from build123d import *

# Parameters (mm, degrees)
F1_DEPTH  = 63.5
F3_DEPTH  = 7.9375
F5_DEPTH  = 7.9375
F7_DEPTH  = 7.9375
F8_R      = 6.35
F9_R      = 9.92251
F10_DEPTH = 88.901
F11_R     = 10.3251
F12_DEPTH = 7.9385


with BuildPart() as f1:
    # F0 (on Right) → F1 (new body)
    with BuildSketch(Plane.YZ):
        with BuildLine():
            Line((-36.5125, 44.45), (-44.45, 44.45))
            Line((-44.45, 44.45), (-44.45, 12.7))
            ThreePointArc((-44.45, 12.7), (-40.7302561211, 3.7197438789), (-31.75, 0))
            Line((-31.75, 0), (0, 0))
            Line((0, 0), (0, 7.9375))
            Line((0, 7.9375), (-31.75, 7.9375))
            ThreePointArc((-31.75, 7.9375), (-35.1175960454, 9.3324039546), (-36.5125, 12.7))
            Line((-36.5125, 12.7), (-36.5125, 44.45))
        make_face()
        with BuildLine():
            Line((0, 7.9375), (0, 0))
            Line((0, 0), (31.75, 0))
            ThreePointArc((31.75, 0), (40.7302561211, 3.7197438789), (44.45, 12.7))
            Line((44.45, 12.7), (44.45, 44.45))
            Line((44.45, 44.45), (36.5125, 44.45))
            Line((36.5125, 44.45), (36.5125, 12.7))
            ThreePointArc((36.5125, 12.7), (35.1175960454, 9.3324039546), (31.75, 7.9375))
            Line((31.75, 7.9375), (0, 7.9375))
        make_face()
    extrude(amount=F1_DEPTH)

    # F2 (on face) → F3 (join, through all)
    with BuildSketch(Plane.XZ.offset(44.45)):
        with BuildLine():
            Line((0, 44.45), (63.5, 44.45))
            ThreePointArc((63.5, 44.45), (31.75, 76.2), (0, 44.45))
        make_face()
    extrude(amount=-F3_DEPTH)

    # F4 (on face) → F5 (join, through all)
    with BuildSketch(Plane(origin=(0, 44.45, 0), x_dir=(-1, 0, 0), z_dir=(0, 1, 0))):
        with BuildLine():
            ThreePointArc((0, 44.45), (-31.75, 76.2), (-63.5, 44.45))
            Line((-63.5, 44.45), (0, 44.45))
        make_face()
    extrude(amount=-F5_DEPTH)

    # F6 (on face) → F7 (join, through all)
    with BuildSketch(Plane(origin=(0, 0, 0), x_dir=(1, 0, 0), z_dir=(0, 0, -1))):
        with BuildLine():
            Line((63.5, 22.225), (63.5, -22.225))
            Line((63.5, -22.225), (117.475, -22.225))
            ThreePointArc((117.475, -22.225), (133.1904482119, -15.7154482119), (139.7, 0))
            ThreePointArc((139.7, 0), (133.1904482119, 15.7154482119), (117.475, 22.225))
            Line((117.475, 22.225), (63.5, 22.225))
        make_face()
    extrude(amount=-F7_DEPTH)

    # F8
    f8_edges = [f1.edges().sort_by_distance(p)[0] for p in [
        (63.5, -22.225, 3.96875),
        (63.5, 22.225, 3.96875),
    ]]
    fillet(f8_edges, radius=F8_R)

    # F9 (on face) → F10 (cut, through all)
    with BuildSketch(Plane.XZ.offset(44.45)):
        with Locations((31.75, 44.45)):
            Circle(F9_R)
    extrude(amount=-F10_DEPTH, mode=Mode.SUBTRACT)

    # F11 (on face) → F12 (cut, through all)
    with BuildSketch(Plane.XY.offset(7.9375)):
        with Locations((117.475, 0)):
            Circle(F11_R)
        with Locations((79.375, 0)):
            Circle(F11_R)
    extrude(amount=-F12_DEPTH, mode=Mode.SUBTRACT)


solid = f1.part
Read the model definition and answer for the solid it produces. Units are mm, in the model's axes. A direction names the side the tool comes from. Give positions to 0.01 mm unless a question says otherwise; leave off trailing zeros. Write each loop counter-clockwise with the first axis right and the second up, starting at its lowest first coordinate (ties: lowest second). Pieces come first, ordered by that corner, then holes. Notation, with made-up numbers: (60, -7) - (80, -7) arc R23 ccw to (80, 21) - close; hole circle Ø4 at (69, 56.5). An arc over 180 degrees is marked (long way). Return JSON: item names as keys, results as strings.
Q1. A cutting plane is placed at B-B, the plane x = 31.75. Count the separate pieces of the cut face and the enclosed holes in it, and give its area (3 significant figures).
Reply:
{"separate pieces": "3", "enclosed holes": "0", "area": "1,410 mm²"}
Q2. For a pull along Y with two mould halves and no side action, classify faces 1 (the face through (32, 44.45, 31)), 2 (the face through (31, -41, 4)), 3 (the face through (89.223, 3.101, 4.024)), 4 (the face through (31.052, 40.537, 76.192)) as released by +Y, released by -Y, zero draft, split by the parting line, or undercut.
Reply:
{"face 1": "released by +Y", "face 2": "released by -Y", "face 3": "undercut", "face 4": "zero draft"}
Q3. A cutting plane is placed at C-C, the plane z = 36.5. Determine the outline of the cut face in (x, y).
Reply:
{"outline": "(0, -44.45) - (25.81, -44.45) - (25.81, -36.51) - (0, -36.51) - close; (0, 36.51) - (25.81, 36.51) - (25.81, 44.45) - (0, 44.45) - close; (37.69, -44.45) - (63.5, -44.45) - (63.5, -36.51) - (37.69, -36.51) - close; (37.69, 36.51) - (63.5, 36.51) - (63.5, 44.45) - (37.69, 44.45) - close"}
Q4. A cutting plane is placed at D-D, the plane x = 84. Determine the outline of the cut face in (y, z) (1 decimal).
Reply:
{"outline": "(-22.2, 0) - (-9.2, 0) - (-9.2, 7.9) - (-22.2, 7.9) - close; (9.2, 0) - (22.2, 0) - (22.2, 7.9) - (9.2, 7.9) - close"}
Q5. Given P1, Ø18.5, axis at x = 79.375, y = 0, coming from the -Z side; P2, Ø5, axis at x = 95.5, y = -8, coming from the +Z side; P3, Ø12.5, axis at y = -35, z = 28.5, coming from the +X side; P4, Ø8.5, axis at x = 86, z = 4, coming from the +Y side (3 decimals), each flat-ended and moving along its own axis, determine where each tip first touches the part or whether it passes through.
Reply:
{"P1": "through", "P2": "z = 7.94", "P3": "x = 63.5", "P4": "y = 22.225"}
Q6. Consider line 1 along Y through (x, z) = (19.5, 23); line 2 along X through (y, z) = (-7, 4); line 3 along X through (y, z) = (41, 44). Determine where each line is inside the solid, lowest interval first. Write a range as [from, to].
Reply:
{"line 1": "[-44.45, -36.51], [36.51, 44.45]", "line 2": "[0, 71.79], [86.96, 109.89], [125.06, 138.57]", "line 3": "[0, 21.84], [41.66, 63.5]"}
Q7. A cutting plane is placed at A-A, the plane z = 26. Determine the outline of the cut face in (x, y), and give its area (3 significant figures).
Reply:
{"outline": "(0, -44.45) - (63.5, -44.45) - (63.5, -36.51) - (0, -36.51) - close; (0, 36.51) - (63.5, 36.51) - (63.5, 44.45) - (0, 44.45) - close", "area": "1,010 mm²"}
Q8. For faces 5 (the face through (63.5, -38, 23)), 6 (the face through (63.5, 38, 23)), 7 (the face through (24, -36.512, 38)), determine the directions among +Z, -Z, +X, -X, +Y, -Y from which every point of the face is accessible in a straight line to the end or side of a thin tool.
Reply:
{"face 5": "+Z, -Z, +X, -Y", "face 6": "+Z, -Z, +X, +Y", "face 7": "+Z, +X, -X"}
